Autodesk Inventor part; units mm, degrees
ref_plane "YZ Plane" through (0, 0, 0) normal (1, 0, 0) x (0, 1, 0)
ref_plane "XZ Plane" through (0, 0, 0) normal (0, 1, 0) x (-1, 0, 0)
ref_plane "XY Plane" through (0, 0, 0) normal (0, 0, 1) x (1, 0, 0)
sketch "Skizze1" plane through (0, 0, 0) normal (0, 1, 0) x (-1, 0, 0)
  line L0 (28.5, 22.5) -> (-28.5, 22.5)
  line L1 (-28.5, 22.5) -> (-28.5, -22.5)
  line L2 (-28.5, -22.5) -> (28.5, -22.5)
  line L3 (28.5, -22.5) -> (28.5, 22.5)
  line L4 (-39.9, 0) -> (39.9, 0)
  line L5 (0, -31.5) -> (0, 31.5)
  circle A0 centre (-25.5, 19.5) radius 1.6
  circle A1 centre (25.5, 19.5) radius 1.6
  circle A2 centre (25.5, -19.5) radius 1.6
  circle A3 centre (-25.5, -19.5) radius 1.6
  line L6 (-28.5, 22.5) -> (-22.5, 22.5)
  line L7 (-22.5, 22.5) -> (-22.5, 16.5)
  line L8 (-22.5, 16.5) -> (-28.5, 16.5)
  line L9 (-28.5, 16.5) -> (-28.5, 22.5)
  line L10 (-14.5, 22.5) -> (-22.5, 22.5)
  line L11 (-22.5, 22.5) -> (-22.5, 16.5)
  line L12 (-22.5, 16.5) -> (-14.5, 16.5)
  line L13 (-14.5, 16.5) -> (-14.5, 22.5)
  line L14 (-28.5, -22.5) -> (-22.5, -22.5)
  line L15 (-22.5, -22.5) -> (-22.5, -16.5)
  line L16 (-22.5, -16.5) -> (-28.5, -16.5)
  line L17 (-28.5, -16.5) -> (-28.5, -22.5)
  line L18 (28.5, -22.5) -> (22.5, -22.5)
  line L19 (22.5, -22.5) -> (22.5, -16.5)
  line L20 (22.5, -16.5) -> (28.5, -16.5)
  line L21 (28.5, -16.5) -> (28.5, -22.5)
  line L22 (28.5, 22.5) -> (22.5, 22.5)
  line L23 (22.5, 22.5) -> (22.5, 16.5)
  line L24 (22.5, 16.5) -> (28.5, 16.5)
  line L25 (28.5, 16.5) -> (28.5, 22.5)
  point P0 (0, 0)
  dimension "d0" = 57
  dimension "d1" = 45
  dimension "d2" = 3.2
  dimension "d3" = 3.2
  dimension "d4" = 3.2
  dimension "d5" = 3.2
  dimension "d6" = 39
  dimension "d7" = 19.5
  dimension "d8" = 51
  dimension "d9" = 51
  dimension "d10" = 39
  dimension "d11" = 19.5
  dimension "d13" = 3
  dimension "d14" = 25.5
  dimension "d15" = 6
  dimension "d16" = 6
  dimension "d17" = 0
  dimension "d18" = 8
  dimension "d19" = 6
  dimension "d20" = 6
  dimension "d21" = 6
  dimension "d22" = 6
  dimension "d23" = 6
  dimension "d24" = 6
extrude "Extrusion1" add sketch "Skizze1" along normal blind 2 and the other way blind 23 contours L3 L24 L23 L0 | L3 L2 L19 L20 | L7 L8 L1 L0 | L16 L15 L2 L1
extrude "Extrusion2" add sketch "Skizze1" along normal blind 2 contours L23 L24 L3 L4 L5 L0 | L5 L4 L1 L8 L12 L13 L0 | L3 L20 L19 L2 L5 L4 | L5 L2 L15 L16 L1 L4
sketch "Skizze2" plane through (-28.5, -23, 22.5) normal (-1, 0, 0) x (0, 0, 1)
  line L0 (0, 0) -> (0, 25)
  line L1 (-45, 0) -> (-45, 25)
  line L2 (0, 25) -> (-45, 25)
  line L3 (-45, 25) -> (-45, 23)
  line L4 (-45, 23) -> (0, 23)
  line L5 (0, 23) -> (0, 25)
  point P0 (-22.5, 23)
extrude "Extrusion3" add sketch "Skizze2" along normal blind 20
sketch "Skizze4" plane through (0, 0, 0) normal (0, -1, 0) x (1, 0, 0)
  line L0 (-48.5, 22.5) -> (-48.5, -22.5)
  line L1 (-48.5, -22.5) -> (-42.5, -22.5)
  line L2 (-42.5, -22.5) -> (-42.5, -16.5)
  line L3 (-42.5, -16.5) -> (-48.5, -16.5)
  line L4 (-48.5, -16.5) -> (-48.5, -22.5)
  line L5 (-48.5, 22.5) -> (-42.5, 22.5)
  line L6 (-42.5, 22.5) -> (-42.5, 16.5)
  line L7 (-42.5, 16.5) -> (-48.5, 16.5)
  line L8 (-48.5, 16.5) -> (-48.5, 22.5)
  line L9 (22.5, -22.5) -> (-22.5, -22.5)
  line L10 (7.5, -22.5) -> (13.5, -22.5)
  line L11 (13.5, -22.5) -> (13.5, -16.5)
  line L12 (13.5, -16.5) -> (7.5, -16.5)
  line L13 (7.5, -16.5) -> (7.5, -22.5)
  line L14 (28.5, 16.5) -> (28.5, -16.5)
  line L15 (-22.5, 22.5) -> (14.5, 22.5)
  line L16 (13.5, 22.5) -> (7.5, 22.5)
  line L17 (7.5, 22.5) -> (7.5, 16.5)
  line L18 (7.5, 16.5) -> (13.5, 16.5)
  line L19 (13.5, 16.5) -> (13.5, 22.5)
  line L20 (28.5, 16.5) -> (28.5, 22.5)
  point P0 (0, 0)
  dimension "d45" = 6
  dimension "d46" = 6
  dimension "d47" = 6
  dimension "d48" = 6
  dimension "d49" = 6
  dimension "d50" = 6
  dimension "d51" = 15
  dimension "d52" = 6
  dimension "d53" = 6
  dimension "d54" = 15
extrude "Extrusion4" add sketch "Skizze4" along normal blind 5
sketch "Skizze3" plane through (0, 2, 0) normal (0, 1, 0) x (1, 0, 0)
  circle A0 centre (10.5, -19.5) radius 2
  circle A1 centre (10.5, 19.5) radius 2
  line L0 (43.9, 0) -> (-63.9, 0)
  line L1 (28.5, -22.5) -> (28.5, 22.5)
  circle A2 centre (-45.5, -19.5) radius 2
  circle A3 centre (-45.5, 19.5) radius 2
  line L2 (14.5, -22.5) -> (-48.5, -22.5)
  line L3 (28.5, 22.5) -> (-48.5, 22.5)
  point P0 (0, 0)
  dimension "d33" = 4
  dimension "d34" = 4
  dimension "d35" = 39
  dimension "d36" = 19.5
  dimension "d37" = 18
  dimension "d38" = 18
  dimension "d39" = 4
  dimension "d40" = 4
  dimension "d41" = 3
  dimension "d42" = 3
  dimension "d43" = 56
  dimension "d44" = 56
extrude "Extrusion5" cut sketch "Skizze3" against normal blind 6
sketch "Skizze5" plane through (0, -23, 0) normal (0, -1, 0) x (1, 0, 0)
  circle A0 centre (-25.5, 19.5) radius 1.6
  circle A1 centre (-25.5, 19.5) radius 1.6
  line L0 (-28.5, 22.5) -> (-22.5, 22.5)
  line L1 (-22.5, 22.5) -> (-22.5, 16.5)
  line L2 (-22.5, 16.5) -> (-28.5, 16.5)
  line L3 (-28.5, 16.5) -> (-28.5, 22.5)
  line L4 (22.5, 16.5) -> (28.5, 16.5)
  line L5 (22.5, 22.5) -> (28.5, 22.5)
  line L6 (28.5, 16.5) -> (22.5, 16.5)
  line L7 (22.5, 16.5) -> (22.5, 22.5)
  line L8 (22.5, 22.5) -> (28.5, 22.5)
  line L9 (28.5, 22.5) -> (28.5, 16.5)
  circle A2 centre (25.5, 19.5) radius 1.6
  circle A3 centre (25.5, -19.5) radius 1.6
  circle A4 centre (25.5, -19.5) radius 1.6
  line L10 (28.5, -22.5) -> (-48.5, -22.5)
  line L11 (22.5, -16.5) -> (22.5, -22.5)
  line L12 (28.5, -22.5) -> (22.5, -22.5)
  line L13 (22.5, -22.5) -> (22.5, -16.5)
  line L14 (22.5, -16.5) -> (28.5, -16.5)
  line L15 (28.5, -16.5) -> (28.5, -22.5)
  line L16 (-28.5, -16.5) -> (-28.5, -22.5)
  line L17 (-22.5, -22.5) -> (-28.5, -22.5)
  line L18 (-28.5, -22.5) -> (-28.5, -16.5)
  line L19 (-28.5, -16.5) -> (-22.5, -16.5)
  line L20 (-22.5, -16.5) -> (-22.5, -22.5)
  circle A5 centre (-25.5, -19.5) radius 1.6
  circle A6 centre (-25.5, -19.5) radius 1.6
  point P0 (0, 0)
  dimension "d59" = 3.2
  dimension "d60" = 3.2
  dimension "d61" = 3.2
  dimension "d62" = 3.2
  dimension "d63" = 3
  dimension "d64" = 3
extrude "Extrusion6" cut sketch "Skizze5" against normal blind 5
sketch "Skizze6" plane through (0, 2, 0) normal (0, 1, 0) x (1, 0, 0)
  line L0 (-44.5, 15) -> (24.5, 15)
  line L1 (24.5, 15) -> (24.5, -15)
  line L2 (24.5, -15) -> (-44.5, -15)
  line L3 (-44.5, -15) -> (-44.5, 15)
  line L4 (43.9, 0) -> (-63.9, 0)
  line L5 (28.5, -22.5) -> (28.5, 22.5)
  point P0 (0, 0)
  dimension "d67" = 69
  dimension "d68" = 30
  dimension "d69" = 4
extrude "Extrusion7" cut sketch "Skizze6" against normal up to surface (2 mm away)
sketch "Skizze8" plane through (14.5, 0, 22.5) normal (0, 0, 1) x (1, 0, 0)
  line L0 (-63, 2) -> (-63, -5)
  line L1 (10, 0) -> (-59, 0)
  line L2 (-63, 2) -> (0, 2)
  line L3 (0, 2) -> (0, 0)
  line L4 (0, 0) -> (-63, 0)
  line L5 (-63, 0) -> (-63, 2)
  line L6 (8, 0) -> (14, 0)
  line L7 (14, 0) -> (8, 0)
  line L8 (8, 0) -> (8, 2)
  line L9 (8, 2) -> (14, 2)
  line L10 (14, 2) -> (14, 0)
  line L11 (8, 2) -> (14, 2)
  point P0 (-14.5, 0)
  point P1 (-63, 0)
  point P2 (-59, 0)
  point P3 (8, 0)
  dimension "d73" = 63
  dimension "d74" = 6
  dimension "d75" = 0
extrude "Extrusion8" add sketch "Skizze8" along normal blind 2
sketch "Skizze9" plane through (28.5, 2, -22.5) normal (0, 0, -1) x (-1, 0, 0)
  line L0 (0, 0) -> (6, 0)
  line L1 (77, -2) -> (77, -7)
  line L2 (0, 0) -> (77, 0)
  line L3 (77, 0) -> (77, -2)
  line L4 (77, -2) -> (0, -2)
  line L5 (0, -2) -> (0, 0)
  point P0 (28.5, -2)
extrude "Extrusion9" add sketch "Skizze9" along normal blind 2
sketch "Skizze7" plane through (0, 2, 0) normal (0, 1, 0) x (1, 0, 0)
  circle A0 centre (-25.5, -19.5) radius 1.6
  circle A1 centre (-25.5, -19.5) radius 2.75
  circle A2 centre (25.5, -19.5) radius 1.6
  circle A3 centre (25.5, -19.5) radius 2.5
  circle A4 centre (25.5, 19.5) radius 1.6
  circle A5 centre (25.5, 19.5) radius 2.75
  circle A6 centre (-25.5, 19.5) radius 1.6
  circle A7 centre (-25.5, 19.5) radius 2.75
  point P0 (0, 0)
  dimension "d72" = 5.5
  dimension "d80" = 5
  dimension "d81" = 5.5
  dimension "d82" = 5.5
sketch "Skizze10" plane through (28.5, 0, 16.5) normal (1, 0, 0) x (0, 0, -1)
  line L0 (41, 2) -> (-8, 2)
  line L1 (39, 0) -> (41, 0)
  line L2 (-8, 2) -> (41, 2)
  line L3 (41, 2) -> (41, 0)
  line L4 (41, 0) -> (-8, 0)
  line L5 (-8, 0) -> (-8, 2)
  point P0 (16.5, 0)
extrude "Extrusion10" add sketch "Skizze10" along normal blind 2
sketch "Skizze11" plane through (-48.5, -23, 22.5) normal (-1, 0, 0) x (0, 0, 1)
  line L0 (-47, 25) -> (2, 25)
  line L1 (2.0117, 23) -> (-47, 23)
  line L2 (-47, 23) -> (-47, 25)
  line L3 (-47, 25) -> (2.0117, 25)
  line L4 (2.0117, 25) -> (2.0117, 23)
  point P0 (-22.5, 23)
  point P1 (2, 25)
extrude "Extrusion11" add sketch "Skizze11" along normal blind 2
extrude "Extrusion12" cut sketch "Skizze7" against normal blind 4
fillet "Rundung1" radius 4 2 edges at (22.5, -9, 22.5) (22.5, 1, 24.5)
properties part number "Adapter_Spannungswandler"
The listing builds one solid part. Answer for the finished solid, in the listing's coordinates (mm). A direction names the side the tool comes from. Give positions to 0.01 mm unless a question says otherwise; leave off trailing zeros. Write each loop counter-clockwise with the first axis right and the second up, starting at its lowest first coordinate (ties: lowest second). Pieces come first, ordered by that corner, then holes. Notation, with made-up numbers: (17, -26) -> (24, -26) arc R20 cw to (24, -12) -> close; hole circle Ø5 at (9, -17). An arc over 180 degrees is marked (long way). Use one line per item in the form item = value.
1) Section D-D on x = -35 is taken. Write down the section's boundary in (y, z), plus the area to 3 significant figures.
Result:
outline = (0, -24.5) -> (2, -24.5) -> (2, -15) -> (0, -15) -> close; (0, 15) -> (2, 15) -> (2, 24.5) -> (0, 24.5) -> close
area = 38.0 mm²
2) Section C-C on z = 4.5 is taken. Write down the section's boundary in (x, y).
Result:
outline = (-50.5, 0) -> (-44.5, 0) -> (-44.5, 2) -> (-50.5, 2) -> close; (24.5, 0) -> (30.5, 0) -> (30.5, 2) -> (24.5, 2) -> close
3) For a pull along X with two mould halves and no side action, classify faces 1 (the flat face through (-24, -2, 21)), 2 (the flat face through (-46, -5, -19)), 3 (the flat face through (-10, 1, 15)), 4 (the flat face through (-48.5, -2, -19)) as +X half, -X half, draft (parallel to the pull), parting line (faces both ways), or undercut.
Result:
face_1 = undercut
face_2 = draft
face_3 = undercut
face_4 = -X half
4) A tool of negligible diameter and unlimited length cuts with its end or side. For faces 5 (the cylindrical face through (-28.247, 0.028, 19.379)), 6 (the flat face through (14.5, 1, 20)), 7 (the flat face through (13.5, -2, -20)), 8 (the flat face through (30.5, 1, 0)), from which of +Z, -Z, +X, -X, +Y, -Y can it reach the whole face along a straight path? Write none if from no direction.
Result:
face_5 = +Y
face_6 = +Z, +Y, -Y
face_7 = +Z, -Z, -Y
face_8 = +Z, -Z, +X, +Y, -Y
5) Straight lines are drawn through the part: probe 1 along Z at (x, y) = (-25.5, -1.1); probe 2 along X at (y, z) = (-8.5, -19.5); probe 3 along Z at (x, y) = (-25.5, -12). For each, find the intervals that lie inside material, in ascending order.
Result:
probe_1 = -22.5 to -22.25, -16.75 to -16.5, 16.5 to 16.75, 22.25 to 22.5
probe_2 = -28.5 to -27.1, -23.9 to -22.5, 22.5 to 23.9, 27.1 to 28.5
probe_3 = -22.5 to -21.1, -17.9 to -16.5, 16.5 to 17.9, 21.1 to 22.5
6) Section B-B on x = -25.5 is taken. Count the separate pieces of the cut face and the enclosed holes in it, plus the area to 3 significant figures.
Result:
separate_pieces = 4
enclosed_holes = 0
area = 108 mm²
7) Section A-A on y = -16.25 is taken. Write down the section's boundary in (x, z).
Result:
outline = (-28.5, -22.5) -> (-22.5, -22.5) -> (-22.5, -16.5) -> (-28.5, -16.5) -> close; (-28.5, 16.5) -> (-22.5, 16.5) -> (-22.5, 22.5) -> (-28.5, 22.5) -> close; (22.5, -22.5) -> (28.5, -22.5) -> (28.5, -16.5) -> (22.5, -16.5) -> close; (22.5, 16.5) -> (28.5, 16.5) -> (28.5, 22.5) -> (26.5, 22.5) arc R4 ccw to (22.5, 18.5) -> close; hole circle Ø3.2 at (-25.5, -19.5); hole circle Ø3.2 at (-25.5, 19.5); hole circle Ø3.2 at (25.5, -19.5); hole circle Ø3.2 at (25.5, 19.5)
8) Each of these flat-tipped pins is pushed along its axis until it touches: P1, Ø1.2, axis at x = -46, z = 19, coming from the +Y side; P2, Ø6.5, axis at x = -44.5, z = 19, coming from the -Y side; P3, Ø1.8, axis at x = -25, y = -5, coming from the -Z side. Where does it stop, or does it pass through?
Result:
P1 = -4
P2 = -5
P3 = -22.5
